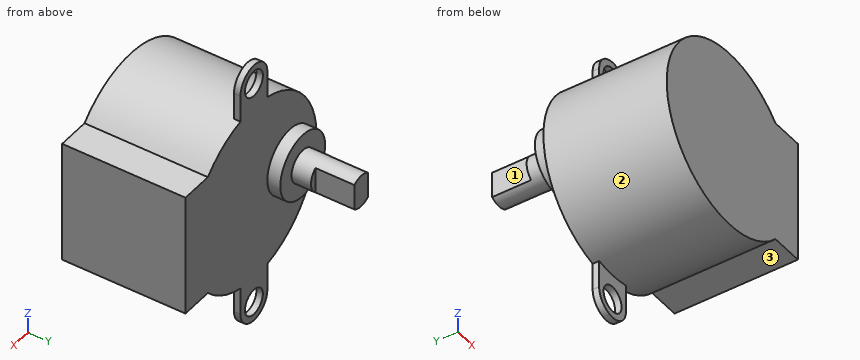
Autodesk Inventor part; units mm, degrees
ref_plane "YZ Plane" through (0, 0, 0) normal (1, 0, 0) x (0, 1, 0)
ref_plane "XZ Plane" through (0, 0, 0) normal (0, 1, 0) x (-1, 0, 0)
ref_plane "XY Plane" through (0, 0, 0) normal (0, 0, 1) x (1, 0, 0)
sketch "Sketch1" plane through (0, 0, 0) normal (0, 1, 0) x (-1, 0, 0)
  circle A0 centre (0, 0) radius 14
  line L0 (-10.2835, 9.5) -> (-15.2835, 9.5)
  line L1 (-15.2835, 9.5) -> (-15.2835, -9.5)
  line L2 (-15.2835, -9.5) -> (-10.2835, -9.5)
  line L3 (-10.2835, -9.5) -> (-10.2835, 9.5)
  point P0 (-10.2835, 0)
  dimension "d0" = 28
  dimension "d3" = 5
  dimension "d4" = 19
extrude "Extrusion1" add sketch "Sketch1" along normal mid plane 19
sketch "Sketch2" plane through (0, 9.5, 0) normal (0, 1, 0) x (1, 0, 0)
  line L0 (0, 0) -> (15.2835, 0) construction
  line L1 (15.2835, -9.5) -> (15.2835, 9.5)
  circle A0 centre (0, 17.9) radius 2
  arc A1 (10.2835, 9.5) -> (10.2835, -9.5) centre (0, 0) ccw
  line L2 (-3, 13.6748) -> (3, 13.6748)
  line L3 (3, 13.6748) -> (3, 17.9)
  line L4 (3, 17.9) -> (-3, 17.9) construction
  line L5 (-3, 17.9) -> (-3, 13.6748)
  arc A2 (3, 17.9) -> (-3, 17.9) centre (0, 17.9) ccw
  circle A3 centre (0, -17.9) radius 2
  line L6 (-3, -13.6748) -> (3, -13.6748)
  line L7 (3, -13.6748) -> (3, -17.9)
  line L8 (3, -17.9) -> (-3, -17.9) construction
  line L9 (-3, -17.9) -> (-3, -13.6748)
  arc A4 (-3, -17.9) -> (3, -17.9) centre (0, -17.9) ccw
  point P0 (0, 14)
  point P1 (0, 13.6748)
  point P2 (0, -14)
  point P3 (0, -13.6748)
  dimension "d5" = 4
  dimension "d6" = 3.9
  dimension "d7" = 3
extrude "Extrusion2" add sketch "Sketch2" against normal blind 1 contours A1 L7 A4 L9 | A1 L5 A2 L3
sketch "Sketch3" plane through (0, 9.5, 0) normal (0, 1, 0) x (1, 0, 0)
  circle A0 centre (-8, 0) radius 5
  arc A1 (-3, 13.6748) -> (-3, -13.6748) centre (0, 0) ccw
  point P0 (-14, 0)
  point P1 (-14, 0)
  dimension "d10" = 10
  dimension "d11" = 6
extrude "Extrusion3" add sketch "Sketch3" along normal blind 2
sketch "Sketch4" plane through (-8, 11.5, 0) normal (0, 1, 0) x (1, 0, 0)
  circle A0 centre (0, 0) radius 2.5
  circle A1 centre (0, 0) radius 5
  point P0 (8, 0)
  dimension "d14" = 5
extrude "Extrusion4" add sketch "Sketch4" along normal blind 9 contours A0
sketch "Sketch5" plane through (-8, 20.5, 0) normal (0, 1, 0) x (1, 0, 0)
  circle A0 centre (0, 0) radius 2.5
  circle A1 centre (0, 0) radius 2.5
  line L0 (1.5, -2) -> (1.5, 2)
  line L1 (0, -2.5) -> (0, 2.5) construction
  line L2 (-1.5, -2) -> (-1.5, 2)
  point P0 (8, 0)
  dimension "d19" = 3
extrude "Extrusion5" cut sketch "Sketch5" against normal blind 6 contours A0 L0 | L2 A0
properties part number "smol stepper"
CAD build for the part. Positions are in the model's coordinates, mm. Face numbers are marked on the shaded views. A direction names the side the tool comes from. Coordinates: 2 decimals unless noted, no trailing zeros. Loops run counter-clockwise (first coordinate to the right, second up) from the corner with the lowest first, then second, coordinate; pieces in that order, holes last. Notation, with made-up numbers: (43.25, 81.25) - (73.25, 81.25) arc R19 cw to (73.25, 116.25) - close; hole circle Ø4 at (81.25, -21.5). An arc over 180 degrees is marked (long way). Return JSON: item names as keys, results as strings.
1. Drop flat-ended pins along their axis: pin 1 (3 mm diameter, centred on x = 4, y = -2.5, fed in from -Z) (3 decimals); pin 2 (1.5 mm diameter, centred on x = -9, y = 9.5, fed in from -Z); pin 3 (10 mm diameter, centred on x = 6, y = -1, fed in from -Z). Give the stop position or say it passes through.
Result:
{"pin 1": "stops at z = -13.775", "pin 2": "stops at z = -11.31", "pin 3": "stops at z = -13.96"}
2. Band-saw the part on C-C (y = 16). Give the cut face in (x, z).
Result:
{"outline": "(-9.5, -2) arc R2.5 ccw to (-6.5, -2) - (-6.5, 2) arc R2.5 ccw to (-9.5, 2) - close"}
3. Band-saw the part on A-A (x = 0). Give the cut face in (y, z), and give its area (3 significant figures).
Result:
{"outline": "(-9.5, -14) - (8.5, -14) - (8.5, -15.9) - (9.5, -15.9) - (9.5, 15.9) - (8.5, 15.9) - (8.5, 14) - (-9.5, 14) - close; (8.5, -20.9) - (9.5, -20.9) - (9.5, -19.9) - (8.5, -19.9) - close; (8.5, 19.9) - (9.5, 19.9) - (9.5, 20.9) - (8.5, 20.9) - close", "area": "538 mm2"}
4. 3-axis set-ups, long thin cutter, end or side, ignore diameter. For the marked faces 1, 2 and 3: which of +Z, -Z, +X, -X, +Y, -Y reach the whole face in a straight line?
Result:
{"face 1": "+Z, -Z, -X, +Y", "face 2": "-Y", "face 3": "-Z, +X, +Y, -Y"}
5. Band-saw the part on D-D (x = -8). Give the cut face in (y, z).
Result:
{"outline": "(-9.5, -11.49) - (9.5, -11.49) - (9.5, -5) - (11.5, -5) - (11.5, -2.5) - (20.5, -2.5) - (20.5, 2.5) - (11.5, 2.5) - (11.5, 5) - (9.5, 5) - (9.5, 11.49) - (-9.5, 11.49) - close"}
6. Probe L1, parallel to Z at x = 0, y = 9.25; L2, parallel to X at y = 9.3, z = -17.9; L3, parallel to X at y = 19, z = -1.5. List the from-to ranges inside material, lowest first. Write a range as from..to.
Result:
{"L1": "z = -20.9..-19.9, -15.9..15.9, 19.9..20.9", "L2": "x = -3..-2, 2..3", "L3": "x = -9.5..-6.5"}
7. Band-saw the part on B-B (z = 0). Give the cut face in (x, y).
Result:
{"outline": "(-14, -9.5) - (15.28, -9.5) - (15.28, 9.5) - (-3, 9.5) - (-3, 11.5) - (-5.5, 11.5) - (-5.5, 14.5) - (-6.5, 14.5) - (-6.5, 20.5) - (-9.5, 20.5) - (-9.5, 14.5) - (-10.5, 14.5) - (-10.5, 11.5) - (-13, 11.5) - (-13, 9.5) - (-14, 9.5) - close"}
